The model under review builds one solid part; all positions refer to its coordinate system, in mm. Face numbers are marked on the shaded views. A direction names the side the tool comes from. Coordinates: 2 decimals unless noted, no trailing zeros. Write each loop counter-clockwise with the first axis right and the second up, starting at its lowest first coordinate (ties: lowest second). Pieces come first, ordered by that corner, then holes. Notation, with made-up numbers: (2.25, -18.75) -> (58.25, -18.75) arc R23 ccw to (58.25, 0.25) -> close; hole circle Ø11 at (12.5, -24). An arc over 180 degrees is marked (long way). Write each question's results on one line, items separated by ' | '.
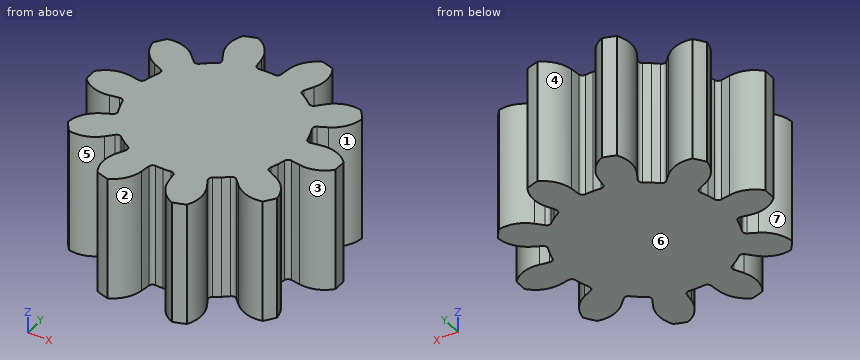
```python
from build123d import *

# Parameters (mm, degrees)
BOSS_EXTRUDE1_DEPTH      = 6
FILLET3_R                = 0.2
FILLET4_R                = 0.2
CIRPATTERN1_COUNT        = 10
FILLET3_OF_CIRPATTERN1_R = 0.2
FILLET4_OF_CIRPATTERN1_R = 0.2


with BuildPart() as part:
    # Sketch1 → Boss-Extrude1 (new body)
    with BuildSketch(Plane.XY):
        with BuildLine():
            Line((0, 0), (3.80266937, -1.235562177))
            ThreePointArc((3.80266937, -1.235562177), (3.87959472, -0.967291603), (3.937619073, -0.694308482))
            Line((3.937619073, -0.694308482), (4.579356052, -0.807464026))
            ThreePointArc((4.579356052, -0.807464026), (5.349965783, -0.745072725), (5.991777209, -0.314015737))
            ThreePointArc((5.991777209, -0.314015737), (6, 0), (5.991777209, 0.314015737))
            ThreePointArc((5.991777209, 0.314015737), (5.349965783, 0.745072725), (4.579356052, 0.807464026))
            Line((4.579356052, 0.807464026), (3.937619073, 0.694308482))
            ThreePointArc((3.937619073, 0.694308482), (3.87959472, 0.967291603), (3.80266937, 1.235562177))
            Line((3.80266937, 1.235562177), (0, 0))
        make_face()
    boss_extrude1 = extrude(amount=BOSS_EXTRUDE1_DEPTH)

    # Fillet3
    fillet3_edges = [part.edges().sort_by_distance(p)[0] for p in [
        (3.937619073, 0.694308482, 3),
    ]]
    fillet(fillet3_edges, radius=FILLET3_R)

    # Fillet4
    fillet4_edges = [part.edges().sort_by_distance(p)[0] for p in [
        (3.937619073, -0.694308482, 3),
    ]]
    fillet(fillet4_edges, radius=FILLET4_R)

    # CirPattern1: Boss-Extrude1 ×10 about axis
    cirpattern1_axis = Axis((0, 0, 0), (0, 0, 1))
    for i in range(1, CIRPATTERN1_COUNT):
        add(boss_extrude1.rotate(cirpattern1_axis, i * 360 / CIRPATTERN1_COUNT))

    # Fillet3 of CirPattern1
    fillet3_of_cirpattern1_edges = [part.edges().sort_by_distance(p)[0] for p in [
        (2.777496461, 2.876181782, 3),
        (0.556464605, 3.959451399, 3),
        (-1.877117817, 3.530345158, 3),
        (-3.593705034, 1.752767059, 3),
        (-3.937619073, -0.694308482, 3),
        (-2.777496461, -2.876181782, 3),
        (-0.556464605, -3.959451399, 3),
        (1.877117817, -3.530345158, 3),
        (3.593705034, -1.752767059, 3),
    ]]
    fillet(fillet3_of_cirpattern1_edges, radius=FILLET3_OF_CIRPATTERN1_R)

    # Fillet4 of CirPattern1
    fillet4_of_cirpattern1_edges = [part.edges().sort_by_distance(p)[0] for p in [
        (3.593705034, 1.752767059, 3),
        (1.877117817, 3.530345158, 3),
        (-0.556464605, 3.959451399, 3),
        (-2.777496461, 2.876181782, 3),
        (-3.937619073, 0.694308482, 3),
        (-3.593705034, -1.752767059, 3),
        (-1.877117817, -3.530345158, 3),
        (0.556464605, -3.959451399, 3),
        (2.777496461, -2.876181782, 3),
    ]]
    fillet(fillet4_of_cirpattern1_edges, radius=FILLET4_OF_CIRPATTERN1_R)


solid = part.part
```
Q1. For line 1 (Y direction, x = -4.5, z = 1.3); line 2 (X direction, y = 3.25, z = 1.15); line 3 (Y direction, x = -4.75, z = 5.8), list the stretches that pass through material, from the lowest coordinate up. Write a range as from..to.
Solution:
line 1: -3.8..-2.25, -0.79..0.79, 2.25..3.8 | line 2: -5.03..-3.14, -2.33..2.33, 3.14..5.03 | line 3: -3.67..-2.52, -0.83..0.83, 2.52..3.67
Q2. Machinability: for the marked faces 1, 2, 3 and 4, which of the approach directions +Z, -Z, +X, -X, +Y, -Y give a long, thin tool a straight path to every point of the face, cutting with its end or side? Answer none if there is none.
Solution:
face 1: +Z, -Z, +X | face 2: +Z, -Z, -Y | face 3: +Z, -Z | face 4: +Z, -Z, +Y
Q3. Draft analysis for pull direction Y (two halves, no side actions). For the marked faces 5, 6 and 7, state which applies: pulls with the +Y half, pulls with the -Y half, needs draft (parallel to the pull), parting line crosses it, or undercut.
Solution:
face 5: pulls with the -Y half | face 6: needs draft | face 7: undercut
Q4. Add section A-A (y = 2.25). Write out the cut boundary in (x, z), plus the area to 3 significant figures.
Solution:
outline: (-4.5, 0) -> (4.5, 0) -> (4.5, 6) -> (-4.5, 6) -> close | area: 54.0 mm²
Q5. Clearance check with flat-ended pins moving along their axes: P1, Ø1.5, axis at y = 3, z = 3, coming from the -X side; P2, Ø1, axis at x = 2.5, y = -4, coming from the -Z side; P3, Ø1.5, axis at y = 2.5, z = 2, coming from the +X side. State where each tip first meets the part, or that it passes through.
Solution:
P1: x = -5.03 | P2: z = 0 | P3: x = 5.03
Q6. Add section B-B (x = -3.5). Write out the cut boundary in (y, z).
Solution:
outline: (-3.57, 0) -> (3.57, 0) -> (3.57, 6) -> (-3.57, 6) -> close
